Input: part model. Units: mm. Frame: model coordinates. Face numbers are marked on the shaded views. A direction names the side the tool comes from. Coordinates: 2 decimals unless noted, no trailing zeros. Order: outer loops, then holes, each group sorted by start corner. A loop starts at its lowest first (then second) coordinate and runs counter-clockwise, first axis right, second up. Notation, with made-up numbers: (30, 9) -> (72, 9) arc R4 ccw to (72, 15) -> close; hole circle Ø5 at (55, -38.5). An arc over 180 degrees is marked (long way). Answer as CSV lines item,"result".
from build123d import *

# Parameters (mm, degrees)
SKETCH1_W           = 25
SKETCH1_H           = 52
BOSS_EXTRUDE1_DEPTH = 7
SKETCH2_R           = 0.9
CUT_EXTRUDE1_DEPTH  = 30.685855218
LPATTERN1_COUNT     = 6
LPATTERN1_PITCH     = 8
SKETCH9_R           = 1.875
SKETCH9_R_2         = 1.6
CUT_EXTRUDE3_DEPTH  = 3.5
LPATTERN2_COUNT     = 6
LPATTERN2_PITCH     = 8
CHAMFER2_SIZE       = 4
SKETCH10_W          = 14.9
SKETCH10_H          = 52
CUT_EXTRUDE4_DEPTH  = 2
CHAMFER3_SIZE       = 2
BOSS_EXTRUDE2_DEPTH = 2
BOSS_EXTRUDE3_DEPTH = 4
SKETCH13_R          = 0.75
CUT_EXTRUDE5_DEPTH  = 3
CUT_EXTRUDE6_REACH  = 31.466
SKETCH14_R          = 1.75
CUT_EXTRUDE7_REACH  = 32.22
SKETCH15_R          = 3


# Some blends are built 0.0001 mm under size
with BuildPart() as part:
    # Sketch1 → Boss-Extrude1 (new body)
    with BuildSketch(Plane(origin=(0, 0, 0), x_dir=(1, 0, 0), z_dir=(0, 1, 0))):
        Rectangle(SKETCH1_W, SKETCH1_H)
    extrude(amount=BOSS_EXTRUDE1_DEPTH)

    # Sketch2 → Cut-Extrude1 (cut, through all)
    with BuildSketch(Plane(origin=(0, 7, 0), x_dir=(1, 0, 0), z_dir=(0, 1, 0))):
        with Locations(Location((-10.45, -20, 0), (0, 0, 270))):
            Circle(SKETCH2_R)
        with Locations(Location((10.45, -20, 0), (0, 0, 270))):
            Circle(SKETCH2_R)
    cut_extrude1 = extrude(amount=-CUT_EXTRUDE1_DEPTH, mode=Mode.SUBTRACT)

    # LPattern1: Cut-Extrude1 ×6
    with Locations(*[(0, 0, -i * LPATTERN1_PITCH) for i in range(1, LPATTERN1_COUNT)]):
        add(cut_extrude1, mode=Mode.SUBTRACT)

    # Sketch9 → Cut-Extrude3 (cut)
    with BuildSketch(Plane(origin=(0, 7, 0), x_dir=(1, 0, 0), z_dir=(0, 1, 0))):
        with Locations(Location((-10.45, 20, 0), (0, 0, 270))):
            Circle(SKETCH9_R)
        with Locations(Location((10.45, 20, 0), (0, 0, 270))):
            Circle(SKETCH9_R_2)
    cut_extrude3 = extrude(amount=-CUT_EXTRUDE3_DEPTH, mode=Mode.SUBTRACT)

    # LPattern2: Cut-Extrude3 ×6
    with Locations(*[(0, 0, i * LPATTERN2_PITCH) for i in range(1, LPATTERN2_COUNT)]):
        add(cut_extrude3, mode=Mode.SUBTRACT)

    # Chamfer2
    # the kernel refuses this chamfer: 4 mm, written as the material it takes off along each edge
    with BuildSketch(Plane(origin=(-12.5, 7, -36.286731952), x_dir=(-0.027495876610586487, -0.9996219169112968, 0), z_dir=(0, 0, 1)), Plane(origin=(12.5, 7, 36.286731952), x_dir=(0.027495876610586487, -0.9996219169112968, 0), z_dir=(0, 0, -1))) as chamfer2_piece_1:
        Polygon((CHAMFER2_SIZE * 0.999621916911, CHAMFER2_SIZE * 0.0274958766106), (-CHAMFER2_SIZE * 0.0274958766106, CHAMFER2_SIZE * 0.999621916911), (0, 0), align=None)
    extrude(amount=72.573463904, mode=Mode.SUBTRACT)

    # Sketch10 → Cut-Extrude4 (cut)
    with BuildSketch(Plane.XZ):
        Rectangle(SKETCH10_W, SKETCH10_H)
    extrude(amount=-CUT_EXTRUDE4_DEPTH, mode=Mode.SUBTRACT)

    # Chamfer3
    chamfer3_edges = [part.edges().sort_by_distance(p)[0] for p in [
        (7.45, 2, 0),
        (-7.45, 2, 0),
    ]]
    chamfer(chamfer3_edges, length=CHAMFER3_SIZE - 0.0001)  # a hair under: the kernel refuses the full size

    # Sketch12 → Boss-Extrude2 (add)
    with BuildSketch(Plane(origin=(0, 7, 0), x_dir=(1, 0, 0), z_dir=(0, 1, 0))):
        with BuildLine():
            ThreePointArc((8.5, 6.164414003), (0, 10.5), (-8.5, 6.164414003))
            Line((-8.5, 6.164414003), (-8.5, -6.164414003))
            ThreePointArc((-8.5, -6.164414003), (0, -10.5), (8.5, -6.164414003))
            Line((8.5, -6.164414003), (8.5, 6.164414003))
        make_face()
    extrude(amount=BOSS_EXTRUDE2_DEPTH)

    # Sketch12<3> → Boss-Extrude3 (add)
    with BuildSketch(Plane(origin=(0, 7, 0), x_dir=(1, 0, 0), z_dir=(0, 1, 0))):
        with BuildLine():
            ThreePointArc((8.5, 10.488088482), (0, 13.5), (-8.5, 10.488088482))
            Line((-8.5, 10.488088482), (-8.5, 6.164414003))
            ThreePointArc((-8.5, 6.164414003), (0, 10.5), (8.5, 6.164414003))
            Line((8.5, 6.164414003), (8.5, 10.488088482))
        make_face()
        with BuildLine():
            Line((-8.5, -6.164414003), (-8.5, -10.488088482))
            ThreePointArc((-8.5, -10.488088482), (0, -13.5), (8.5, -10.488088482))
            Line((8.5, -10.488088482), (8.5, -6.164414003))
            ThreePointArc((8.5, -6.164414003), (0, -10.5), (-8.5, -6.164414003))
        make_face()
    extrude(amount=BOSS_EXTRUDE3_DEPTH)

    # Sketch13 → Cut-Extrude5 (cut)
    with BuildSketch(Plane(origin=(0, 9, 0), x_dir=(1, 0, 0), z_dir=(0, 1, 0))):
        with Locations(Location((-5.091168825, 5.091168825, 0), (0, 0, 270))):
            Circle(SKETCH13_R)
        with Locations(Location((5.091168825, 5.091168825, 0), (0, 0, 270))):
            Circle(SKETCH13_R)
        with Locations(Location((5.091168825, -5.091168825, 0), (0, 0, 270))):
            Circle(SKETCH13_R)
        with Locations(Location((-5.091168825, -5.091168825, 0), (0, 0, 270))):
            Circle(SKETCH13_R)
    extrude(amount=-CUT_EXTRUDE5_DEPTH, mode=Mode.SUBTRACT)

    # Sketch14 → Cut-Extrude6 (cut, up to next)
    with BuildSketch(Plane(origin=(0, 6, 0), x_dir=(1, 0, 0), z_dir=(0, 1, 0)), mode=Mode.PRIVATE) as cut_extrude6_sk1:
        with Locations(Location((-5.091168825, 5.091168825, 0), (0, 0, 270))):
            Circle(SKETCH14_R)
    cut_extrude6_tool1 = extrude(cut_extrude6_sk1.sketch, amount=-CUT_EXTRUDE6_REACH, mode=Mode.PRIVATE) & part.part
    # Sketch14 → Cut-Extrude6 (cut, up to next)
    with BuildSketch(Plane(origin=(0, 6, 0), x_dir=(1, 0, 0), z_dir=(0, 1, 0)), mode=Mode.PRIVATE) as cut_extrude6_sk2:
        with Locations(Location((5.091168825, 5.091168825, 0), (0, 0, 270))):
            Circle(SKETCH14_R)
    cut_extrude6_tool2 = extrude(cut_extrude6_sk2.sketch, amount=-CUT_EXTRUDE6_REACH, mode=Mode.PRIVATE) & part.part
    # Sketch14 → Cut-Extrude6 (cut, up to next)
    with BuildSketch(Plane(origin=(0, 6, 0), x_dir=(1, 0, 0), z_dir=(0, 1, 0)), mode=Mode.PRIVATE) as cut_extrude6_sk3:
        with Locations(Location((5.091168825, -5.091168825, 0), (0, 0, 270))):
            Circle(SKETCH14_R)
    cut_extrude6_tool3 = extrude(cut_extrude6_sk3.sketch, amount=-CUT_EXTRUDE6_REACH, mode=Mode.PRIVATE) & part.part
    # Sketch14 → Cut-Extrude6 (cut, up to next)
    with BuildSketch(Plane(origin=(0, 6, 0), x_dir=(1, 0, 0), z_dir=(0, 1, 0)), mode=Mode.PRIVATE) as cut_extrude6_sk4:
        with Locations(Location((-5.091168825, -5.091168825, 0), (0, 0, 270))):
            Circle(SKETCH14_R)
    cut_extrude6_tool4 = extrude(cut_extrude6_sk4.sketch, amount=-CUT_EXTRUDE6_REACH, mode=Mode.PRIVATE) & part.part
    add(cut_extrude6_tool1.solids().sort_by_distance((-5.091169, 6, -5.091169))[0], mode=Mode.SUBTRACT)
    add(cut_extrude6_tool2.solids().sort_by_distance((5.091169, 6, -5.091169))[0], mode=Mode.SUBTRACT)
    add(cut_extrude6_tool3.solids().sort_by_distance((5.091169, 6, 5.091169))[0], mode=Mode.SUBTRACT)
    add(cut_extrude6_tool4.solids().sort_by_distance((-5.091169, 6, 5.091169))[0], mode=Mode.SUBTRACT)

    # Sketch15 → Cut-Extrude7 (cut, up to next)
    with BuildSketch(Plane(origin=(0, 9, 0), x_dir=(1, 0, 0), z_dir=(0, 1, 0)), mode=Mode.PRIVATE) as cut_extrude7_sk1:
        with Locations(Location((0, 0, 0), (0, 0, 270))):
            Circle(SKETCH15_R)
    cut_extrude7_tool1 = extrude(cut_extrude7_sk1.sketch, amount=-CUT_EXTRUDE7_REACH, mode=Mode.PRIVATE) & part.part
    add(cut_extrude7_tool1.solids().sort_by_distance((0, 9, 0))[0], mode=Mode.SUBTRACT)


solid = part.part
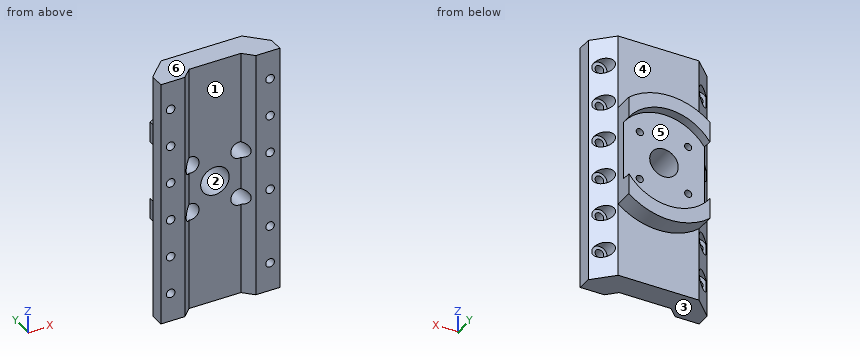
1. Ray query, line 1 along X through (y, z) = (4.9, 4) (3 decimals); line 2 along Y through (x, z) = (-1, 18.5); line 3 along X through (y, z) = (1.2, 4). Return the intervals inside material, ascending.
Findings:
line 1,"x = -8.575 to -6.459, -3.723 to 3.723, 6.459 to 8.85"
line 2,"y = 2 to 7"
line 3,"x = -12.5 to -11.35, -9.55 to -6.46, 6.46 to 9.55, 11.35 to 12.5"
2. Mould query, pull axis Z, two halves, no side actions, for the marked faces 3, 4, 5 and 6. Classes: released by +Z, released by -Z, zero draft, split by the parting line, or undercut.
Findings:
face 3,"released by -Z"
face 4,"zero draft"
face 5,"undercut"
face 6,"released by +Z"
3. Cut plane C-C (x = 1). Return the cut outline in (y, z).
Findings:
outline,"(2, -26) -> (7, -26) -> (7, -13.46) -> (11, -13.46) -> (11, -10.45) -> (9, -10.45) -> (9, -2.83) -> (2, -2.83) -> close; (2, 2.83) -> (9, 2.83) -> (9, 10.45) -> (11, 10.45) -> (11, 13.46) -> (7, 13.46) -> (7, 26) -> (2, 26) -> close"
4. Cut plane D-D (y = 1.5). State how many separate pieces and enclosed holes the cut face has, plus the area to 3 significant figures.
Findings:
separate pieces,"2"
enclosed holes,"12"
area,"643 mm2"
5. Contact query for flat-ended pins moving along their axis: pin 1 (2 mm diameter, centred on y = 8.5, z = -3.5, fed in from -X); pin 2 (2 mm diameter, centred on x = -10.45, z = -4, fed in from -Y); pin 3 (4 mm diameter, centred on x = 10.45, z = -4, fed in from +Y); pin 4 (1.1 mm diameter, centred on x = 10.45, z = 4, fed in from -Y). Output: stop coordinate, or through.
Findings:
pin 1,"stops at x = -8.5"
pin 2,"stops at y = 0"
pin 3,"stops at y = 9"
pin 4,"passes through"
6. Reachability of the marked faces 1 and 2 from +Z, -Z, +X, -X, +Y, -Y: full face, straight path, thin tool, end or side. Return the list, or none.
Findings:
face 1,"+Z, -Z, -Y"
face 2,"+Y, -Y"
7. Cut plane A-A (y = 10). Return the cut outline in (x, z), plus the area to 3 significant figures.
Findings:
outline,"(-8.5, -10.49) arc R13.5 ccw to (8.5, -10.49) -> (8.5, -6.16) arc R10.5 cw to (-8.5, -6.16) -> close; (-8.5, 6.16) arc R10.5 cw to (8.5, 6.16) -> (8.5, 10.49) arc R13.5 ccw to (-8.5, 10.49) -> close"
area,"114 mm2"
